```python
from build123d import *

# Parameters (mm, degrees)
SKETCH1_R           = 2.286
BOSS_EXTRUDE1_DEPTH = 19.05
BOSS_EXTRUDE2_DEPTH = 5.175
SKETCH2_R           = 1.25
SKETCH2_R_2         = 4.365625
CUT_EXTRUDE1_DEPTH  = 5.175
SKETCH4_R           = 2
CUT_EXTRUDE2_DEPTH  = 2


with BuildPart() as part:
    # Sketch1 → Boss-Extrude1 (new body)
    with BuildSketch(Plane.XY):
        Polygon((8.255, 25.368), (8.255, 5.175), (48.895, 5.175), (48.895, 25.368), (57.15, 25.368), (57.15, 0), (0, 0), (0, 25.368), align=None)
        with Locations((4.445, 21.431)):
            Circle(SKETCH1_R, mode=Mode.SUBTRACT)
        with Locations((4.445, 9.112)):
            Circle(SKETCH1_R, mode=Mode.SUBTRACT)
        with Locations((52.705, 9.112)):
            Circle(SKETCH1_R, mode=Mode.SUBTRACT)
        with Locations((52.705, 21.431)):
            Circle(SKETCH1_R, mode=Mode.SUBTRACT)
    extrude(amount=BOSS_EXTRUDE1_DEPTH)

    # Sketch3 → Boss-Extrude2 (add)
    with BuildSketch(Plane.XZ):
        Polygon((25.4, 29.21), (31.75, 29.21), (44.45, 19.05), (44.45, 0), (31.75, -10.16), (25.4, -10.16), (12.7, 0), (12.7, 19.05), align=None)
    extrude(amount=-BOSS_EXTRUDE2_DEPTH)

    # Sketch2 → Cut-Extrude1 (cut)
    with BuildSketch(Plane.XZ):
        with Locations((36.5750114, 9.525)):
            Circle(SKETCH2_R)
        with Locations((39.5750054, 9.525)):
            Circle(SKETCH2_R)
        with Locations((42.5749994, 9.525)):
            Circle(SKETCH2_R)
        with Locations((45.5749934, 9.525)):
            Circle(SKETCH2_R)
        with Locations((28.575, 1.5249886)):
            Circle(SKETCH2_R)
        with Locations((28.575, -1.4750054)):
            Circle(SKETCH2_R)
        with Locations((28.575, -4.4749994)):
            Circle(SKETCH2_R)
        with Locations((28.575, -7.4749934)):
            Circle(SKETCH2_R)
        with Locations((20.5749886, 9.525)):
            Circle(SKETCH2_R)
        with Locations((17.5749946, 9.525)):
            Circle(SKETCH2_R)
        with Locations((14.5750006, 9.525)):
            Circle(SKETCH2_R)
        with Locations((11.5750066, 9.525)):
            Circle(SKETCH2_R)
        with Locations((28.575, 17.5250114)):
            Circle(SKETCH2_R)
        with Locations((28.575, 20.5250054)):
            Circle(SKETCH2_R)
        with Locations((28.575, 23.5249994)):
            Circle(SKETCH2_R)
        with Locations((28.575, 26.5249934)):
            Circle(SKETCH2_R)
        with Locations((28.575, 9.525)):
            Circle(SKETCH2_R_2)
    extrude(amount=-CUT_EXTRUDE1_DEPTH, mode=Mode.SUBTRACT)

    # Sketch4 → Cut-Extrude2 (cut)
    with BuildSketch(Plane(origin=(0, 5.175, 0), x_dir=(1, 0, 0), z_dir=(0, 1, 0))):
        with Locations((28.575, 1.4750054)):
            Circle(SKETCH4_R)
        with Locations((28.575, 7.4749934)):
            Circle(SKETCH4_R)
        with Locations((11.5750066, -9.525)):
            Circle(SKETCH4_R)
        with Locations((17.5749946, -9.525)):
            Circle(SKETCH4_R)
        with Locations((36.5750114, -9.525)):
            Circle(SKETCH4_R)
        with Locations((28.575, -20.5250054)):
            Circle(SKETCH4_R)
        with Locations((45.5749934, -9.525)):
            Circle(SKETCH4_R)
        with Locations((28.575, -26.5249934)):
            Circle(SKETCH4_R)
    extrude(amount=-CUT_EXTRUDE2_DEPTH, mode=Mode.SUBTRACT)


solid = part.part
```
Input: part model. Units: mm. Frame: model coordinates. A direction names the side the tool comes from. Coordinates: 2 decimals unless noted, no trailing zeros. Order: outer loops, then holes, each group sorted by start corner. A loop starts at its lowest first (then second) coordinate and runs counter-clockwise, first axis right, second up. Notation, with made-up numbers: (-10, -10.5) - (47, -10.5) arc R25 cw to (47, 27.5) - close; hole circle Ø1 at (65, 81.25). An arc over 180 degrees is marked (long way). Put each result on its own line as item: value.
1. Cut plane C-C on z = 4. Return the cut outline in (x, y) (3 decimals).
Report:
outline: (0, 0) - (57.15, 0) - (57.15, 25.368) - (48.895, 25.368) - (48.895, 5.175) - (8.255, 5.175) - (8.255, 25.368) - (0, 25.368) - close; hole circle Ø4.572 at (4.445, 9.112); hole circle Ø4.572 at (4.445, 21.431); hole circle Ø4.572 at (52.705, 9.112); hole circle Ø4.572 at (52.705, 21.431)
2. Cut plane D-D on y = 1.75. State how many separate pieces and enclosed holes the cut face has, then the cut area to 3 significant figures.
Report:
separate pieces: 1
enclosed holes: 17
area: 1,340 mm2
3. Reachability of faces 1 (the face through (17.61, 4.189, 7.525)), 2 (the face through (8.255, 15, 9)), 3 (the face through (19.14, 2.55, -5.15)) from +Z, -Z, +X, -X, +Y, -Y: full face, straight path, thin tool, end or side. Return the list, or none.
Report:
face 1: +Y
face 2: +Z, -Z, +Y
face 3: -Z, -X, +Y, -Y
4. Draft query along X for faces 4 (the face through (52, 13, 19.05)), 5 (the face through (18.96, 2.55, 24.06)), 6 (the face through (30.575, 4.189, -1.44)). Return one class per face: pulls with the +X half, pulls with the -X half, needs draft (parallel to the pull), parting line crosses it, or undercut.
Report:
face 4: needs draft
face 5: pulls with the -X half
face 6: undercut
5. Line query: line 1 along Y through (x, z) = (23, 24) (3 decimals); line 2 along X through (y, z) = (18, 15.5) (3 decimals); line 3 along Z through (x, y) = (8, 9.5). Output: solid intervals per line, ascending.
Report:
line 1: y = 0 to 5.175
line 2: x = 0 to 8.255, 48.895 to 57.15
line 3: z = 0 to 19.05
6. Contact query for flat-ended pins moving along their axis: pin 1 Ø4 at (y, z) = (11, 3) entering from -X; pin 2 Ø5.5 at (x, y) = (4.445, 9.112) entering from -Z; pin 3 Ø1.5 at (x, z) = (45.57, 9.52) entering from -Y; pin 4 Ø12 at (x, z) = (31.5, 21) entering from +Y (3 decimals). Output: stop coordinate, or through.
Report:
pin 1: stops at x = 0
pin 2: stops at z = 0
pin 3: passes through
pin 4: stops at y = 5.175
7. Cut plane B-B on x = 5.5. Return the cut outline in (y, z), then the cut area to 3 significant figures.
Report:
outline: (0, 0) - (7.08, 0) - (7.08, 19.05) - (0, 19.05) - close; (11.14, 0) - (19.4, 0) - (19.4, 19.05) - (11.14, 19.05) - close; (23.46, 0) - (25.37, 0) - (25.37, 19.05) - (23.46, 19.05) - close
area: 329 mm2
8. Cut plane A-A on y = 17.75. Return the cut outline in (x, z) (3 decimals).
Report:
outline: (0, 0) - (8.255, 0) - (8.255, 19.05) - (0, 19.05) - close; (48.895, 0) - (57.15, 0) - (57.15, 19.05) - (48.895, 19.05) - close
